Read the model definition and answer for the solid it produces. Units are mm, in the model's axes. Coordinates: 2 decimals unless noted, no trailing zeros. Write each loop counter-clockwise with the first axis right and the second up, starting at its lowest first coordinate (ties: lowest second). Pieces come first, ordered by that corner, then holes.
from build123d import *

# Parameters (mm, degrees)
SKETCH1_W           = 402
SKETCH1_H           = 50
SKETCH1_R           = 6
SKETCH1_R_2         = 1.8
SKETCH1_R_3         = 11
SKETCH1_R_4         = 2.6
BOSS_EXTRUDE1_DEPTH = 8


with BuildPart() as part:
    # Sketch1 → Boss-Extrude1 (new body)
    with BuildSketch(Plane.XY):
        Rectangle(SKETCH1_W, SKETCH1_H)
        with Locations((-178, 0)):
            Circle(SKETCH1_R, mode=Mode.SUBTRACT)
        with Locations((168, 0)):
            Circle(SKETCH1_R_2, mode=Mode.SUBTRACT)
        Circle(SKETCH1_R_3, mode=Mode.SUBTRACT)
        with Locations((-188, 0)):
            Circle(SKETCH1_R_2, mode=Mode.SUBTRACT)
        with Locations((-168, 0)):
            Circle(SKETCH1_R_2, mode=Mode.SUBTRACT)
        with Locations((188, 0)):
            Circle(SKETCH1_R_2, mode=Mode.SUBTRACT)
        with Locations((178, 0)):
            Circle(SKETCH1_R, mode=Mode.SUBTRACT)
        with Locations((0, 17)):
            Circle(SKETCH1_R_4, mode=Mode.SUBTRACT)
        with Locations((-40, 17)):
            Circle(SKETCH1_R_4, mode=Mode.SUBTRACT)
        with Locations((-80, 17)):
            Circle(SKETCH1_R_4, mode=Mode.SUBTRACT)
        with Locations((-120, 17)):
            Circle(SKETCH1_R_4, mode=Mode.SUBTRACT)
        with Locations((-160, 17)):
            Circle(SKETCH1_R_4, mode=Mode.SUBTRACT)
        with Locations((40, 17)):
            Circle(SKETCH1_R_4, mode=Mode.SUBTRACT)
        with Locations((80, 17)):
            Circle(SKETCH1_R_4, mode=Mode.SUBTRACT)
        with Locations((120, 17)):
            Circle(SKETCH1_R_4, mode=Mode.SUBTRACT)
        with Locations((160, 17)):
            Circle(SKETCH1_R_4, mode=Mode.SUBTRACT)
    extrude(amount=BOSS_EXTRUDE1_DEPTH)


solid = part.part
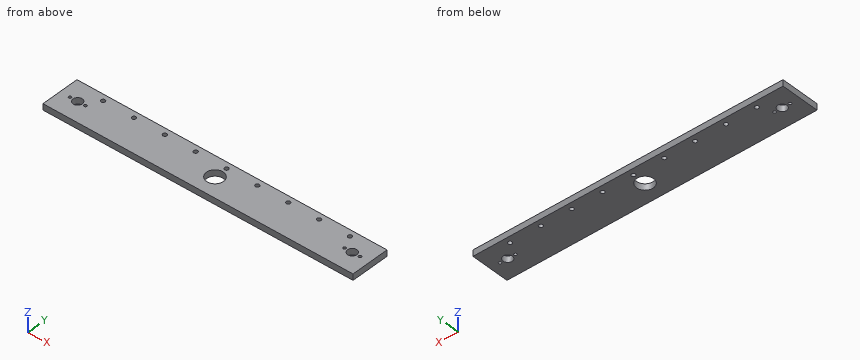
Item 1: Find the intervals of material crossed by probe 1 along Y at (x, z) = (-120, 5.5); probe 2 along Y at (x, z) = (0, 4); probe 3 along X at (y, z) = (4, 4.25), in increasing order.
Item 2: Given pin 1 (9.5 mm diameter, centred on x = -178, y = 0, fed in from +Z), flat-ended and moving along its own axis, determine where the tip first touches the part or whether it passes through.
Item 3: The part is cut by section B-B (z = 4). State how many separate pieces and enclosed holes the cut face has, and give its area (3 significant figures).
Item 4: The part is cut by section A-A (x = 178). Give the vertices of the cut face in (y, z), and give its area (3 significant figures).
Answer:
1. probe 1: y = -25 to 14.4, 19.6 to 25
1. probe 2: y = -25 to -11, 11 to 14.4, 19.6 to 25
1. probe 3: x = -201 to -182.47, -173.53 to -10.25, 10.25 to 173.53, 182.47 to 201
2. pin 1: passes through
3. separate pieces: 1
3. enclosed holes: 16
3. area: 19,300 mm2
4. outline: (-25, 0) - (-6, 0) - (-6, 8) - (-25, 8) - close; (6, 0) - (25, 0) - (25, 8) - (6, 8) - close
4. area: 304 mm2
